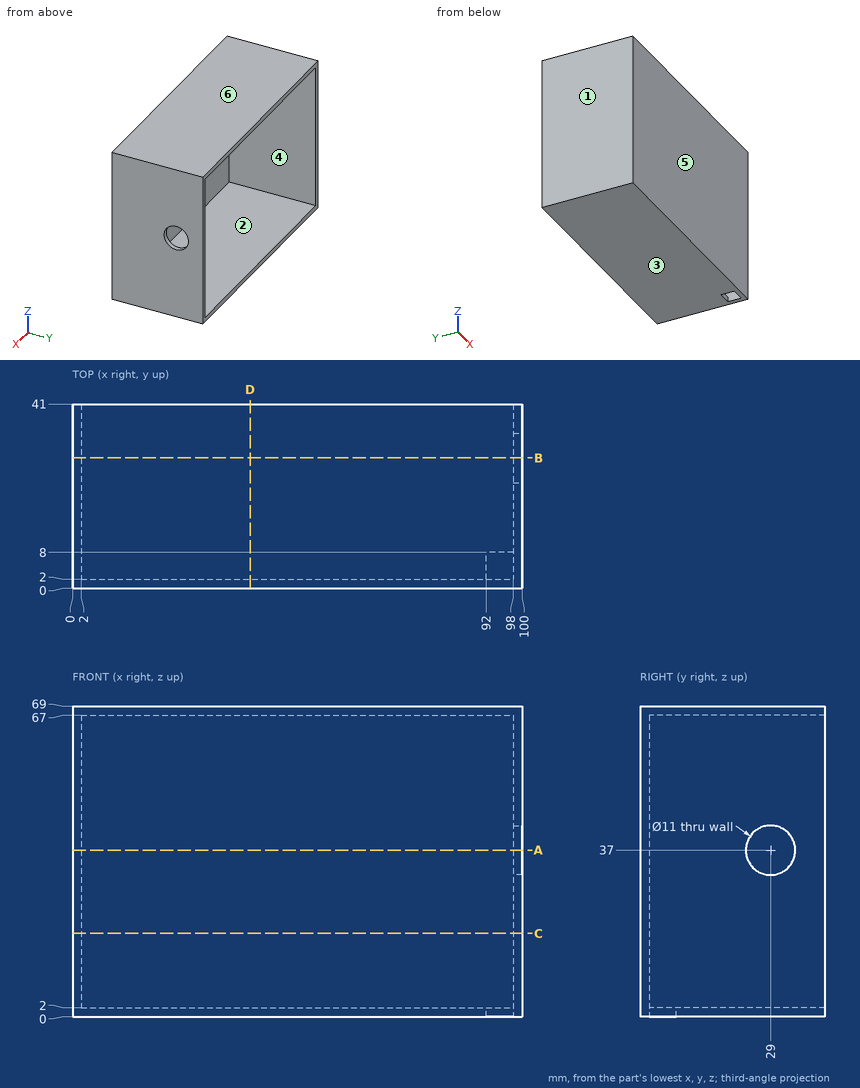
For this review, use the dimensioned drawing (mm, ordinates from the lowest corner) and the shaded views. A direction names the side the tool comes from. Coordinates: 2 decimals unless noted, no trailing zeros. Loops run counter-clockwise (first coordinate to the right, second up) from the corner with the lowest first, then second, coordinate; pieces in that order, holes last.
1. Mouldability with a two-part tool opening along Z and no side actions: class the marked faces 3, 4, 5 and 6 as +Z half, -Z half, draft (parallel to the pull), parting line (faces both ways), or undercut.
2. For the marked faces 1 and 2, list the 3-axis set-ups (+Z, -Z, +X, -X, +Y, -Y) from which the entire face can be reached by the end or side of a thin tool; tool diameter is ignored.
3. For line 1 (Z direction, x = 43.5, y = 29); line 2 (X direction, y = 10, z = 18.5); line 3 (Y direction, x = 99.05, z = 37), list the stretches that pass through material, from the lowest coordinate up.
4. Add section B-B, the plane y = 29. Give the boundary of the cut face in (x, z), then the cut area to 3 significant figures.
5. Add section C-C, the plane z = 18.5. Give the boundary of the cut face in (x, y), then the cut area to 3 significant figures.
6. Add section D-D, the plane x = 39.5. Give the boundary of the cut face in (y, z).
7. Insertion check: P1, Ø1.5, axis at x = 62, y = 13, coming from the -Z side; P2, Ø1, axis at x = 68.5, z = 29.5, coming from the +Y side. Each pin has a flat end and moves straight along its axis. Give the tip position at first contact, or say it passes through.
8. Add section A-A, the plane z = 37. Give the boundary of the cut face in (x, y), then the cut area to 3 significant figures.
Result:
1. face 3: -Z half
1. face 4: undercut
1. face 5: draft
1. face 6: +Z half
2. face 1: +Z, -Z, -X, +Y, -Y
2. face 2: +Y
3. line 1: z = 0 to 2, 67 to 69
3. line 2: x = 0 to 2, 98 to 100
3. line 3: y = 0 to 23.5, 34.5 to 41
4. outline: (0, 0) - (100, 0) - (100, 31.5) - (98, 31.5) - (98, 2) - (2, 2) - (2, 67) - (98, 67) - (98, 42.5) - (100, 42.5) - (100, 69) - (0, 69) - close
4. area: 638 mm2
5. outline: (0, 0) - (100, 0) - (100, 41) - (98, 41) - (98, 2) - (2, 2) - (2, 41) - (0, 41) - close
5. area: 356 mm2
6. outline: (0, 0) - (41, 0) - (41, 2) - (2, 2) - (2, 67) - (41, 67) - (41, 69) - (0, 69) - close
7. P1: stops at z = 0
7. P2: stops at y = 2
8. outline: (0, 0) - (100, 0) - (100, 23.5) - (98, 23.5) - (98, 2) - (2, 2) - (2, 41) - (0, 41) - close; (98, 34.5) - (100, 34.5) - (100, 41) - (98, 41) - close
8. area: 334 mm2
